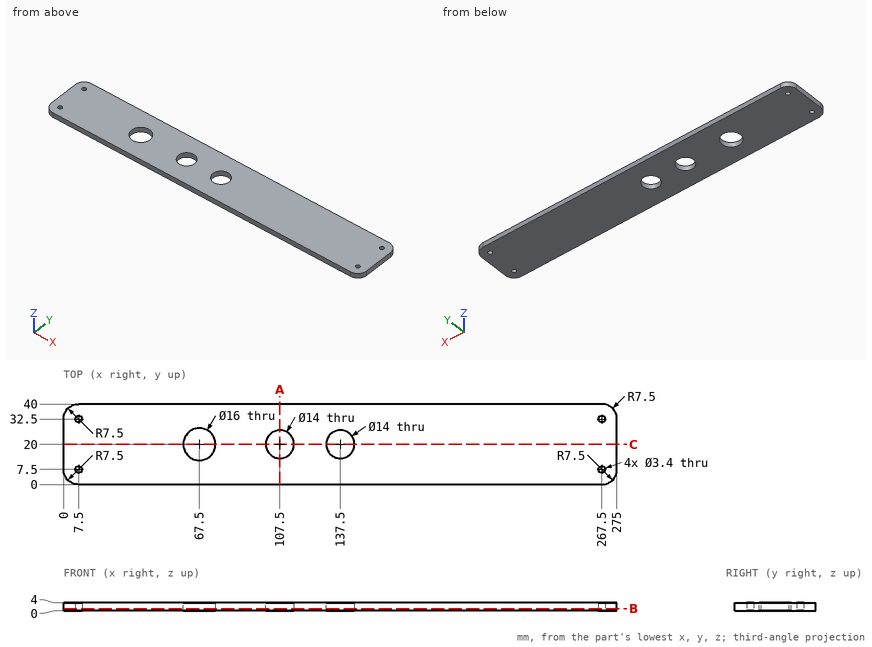
Geometry: see drawing. Coordinates: mm, zero at the bounding-box minimum. Give positions to 0.01 mm unless a question says otherwise; leave off trailing zeros. Order: outer loops, then holes, each group sorted by start corner. A loop starts at its lowest first (then second) coordinate and runs counter-clockwise, first axis right, second up. Notation, with made-up numbers: (86, -37.5) -> (102, -37.5) arc R23 cw to (102, -8.5) -> close; hole circle Ø11 at (28.25, 8.25). An arc over 180 degrees is marked (long way). Write each question's results on one line, items separated by ' | '. Start each with the question number.
1) Section C-C (y = 20). Return loops of the section in (x, z).
2) Section B-B (z = 1). Return loops of the section in (x, y), then the cut area to 3 significant figures.
3) Section A-A (x = 107.5). Return loops of the section in (y, z), then the cut area to 3 significant figures.
4) First-contact query: pin 1 (9.5 mm diameter, centred on x = 67.5, y = 20, fed in from -Z). Flat tip, straight axial feed; report the tip coordinate or a pass-through.
5) Line query: line 1 (Y direction, x = 267.5, z = 1.8); line 2 (Y direction, x = 107.5, z = 1.65); line 3 (X direction, y = 33.5, z = 2.3). Output: solid intervals per line, ascending. Write a range as from..to.
Calculated:
1) outline: (0, 0) -> (59.5, 0) -> (59.5, 4) -> (0, 4) -> close; (75.5, 0) -> (100.5, 0) -> (100.5, 4) -> (75.5, 4) -> close; (114.5, 0) -> (130.5, 0) -> (130.5, 4) -> (114.5, 4) -> close; (144.5, 0) -> (275, 0) -> (275, 4) -> (144.5, 4) -> close
2) outline: (0, 7.5) arc R7.5 ccw to (7.5, 0) -> (267.5, 0) arc R7.5 ccw to (275, 7.5) -> (275, 32.5) arc R7.5 ccw to (267.5, 40) -> (7.5, 40) arc R7.5 ccw to (0, 32.5) -> close; hole circle Ø3.4 at (7.5, 7.5); hole circle Ø3.4 at (7.5, 32.5); hole circle Ø16 at (67.5, 20); hole circle Ø14 at (107.5, 20); hole circle Ø14 at (137.5, 20); hole circle Ø3.4 at (267.5, 7.5); hole circle Ø3.4 at (267.5, 32.5) | area: 10,400 mm2
3) outline: (0, 0) -> (13, 0) -> (13, 4) -> (0, 4) -> close; (27, 0) -> (40, 0) -> (40, 4) -> (27, 4) -> close | area: 104 mm2
4) pin 1: through
5) line 1: 0..5.8, 9.2..30.8, 34.2..40 | line 2: 0..13, 27..40 | line 3: 0.07..6.13, 8.87..266.13, 268.87..274.93
